```python
from build123d import *

# Parameters (mm, degrees)
SKETCH2_R           = 1.5
BOSS_EXTRUDE1_DEPTH = 45
CHAMFER1_SIZE       = 0.3
SKETCH6_W           = 3
SKETCH6_H           = 2.75
CUT_EXTRUDE1_DEPTH  = 1.6
SKETCH8_R           = 1.493375673
CUT_EXTRUDE2_DEPTH  = 1
CUT_EXTRUDE2_TAPER  = 45


with BuildPart() as part:
    # Sketch2 → Boss-Extrude1 (new body)
    with BuildSketch(Plane(origin=(0, 0, 0), x_dir=(0, 0, -1), z_dir=(1, 0, 0))):
        Circle(SKETCH2_R)
    extrude(amount=-BOSS_EXTRUDE1_DEPTH)

    # Chamfer1
    chamfer1_edges = [part.edges().sort_by_distance(p)[0] for p in [
        (0, 0, 1.5),
    ]]
    chamfer(chamfer1_edges, length=CHAMFER1_SIZE)

    # Sketch6 → Revolve1 (revolve)
    with BuildSketch(Plane.XY):
        with Locations((-46.5, 1.375)):
            Rectangle(SKETCH6_W, SKETCH6_H)
    revolve(axis=Axis((-45, 0, 0), (1, 0, 0)))

    # Sketch7 → Cut-Extrude1 (cut)
    with BuildSketch(Plane.ZY.offset(48)):
        Polygon((0, 1.443375673), (-1.25, 0.721687836), (-1.25, -0.721687836), (0, -1.443375673), (1.25, -0.721687836), (1.25, 0.721687836), align=None)
    extrude(amount=-CUT_EXTRUDE1_DEPTH, mode=Mode.SUBTRACT)

    # Sketch8 → Cut-Extrude2 (cut)
    with BuildSketch(Plane.ZY.offset(48)):
        Circle(SKETCH8_R)
    extrude(amount=-CUT_EXTRUDE2_DEPTH, taper=CUT_EXTRUDE2_TAPER, mode=Mode.SUBTRACT)


solid = part.part
```
The listing builds one solid part. Answer for the finished solid, in the listing's coordinates (mm). A direction names the side the tool comes from. Coordinates: 2 decimals unless noted, no trailing zeros. Loops run counter-clockwise (first coordinate to the right, second up) from the corner with the lowest first, then second, coordinate; pieces in that order, holes last. Notation, with made-up numbers: (8.25, -39.5) -> (28.25, -39.5) arc R22 cw to (28.25, -31.5) -> close; hole circle Ø6 at (45, -13.75). An arc over 180 degrees is marked (long way). Return JSON: item names as keys, results as strings. Group by question number.
(1) Determine the mould class of faces 1 (the cylindrical face through (-46.479, -0.596, -2.685)), 2 (the flat face through (-46.4, 0, 0)), 3 (the flat face through (-48, -1.2, -1.2)) for opening direction Y: released by +Y, released by -Y, zero draft, split by the parting line, or undercut.
(2) Which of the six approach directions +Z, -Z, +X, -X, +Y, -Y give full straight-line access (tool end or side, diameter ignored) to faces 4 (the flat face through (-45, -1.2, -1.2)), 5 (the flat face through (0, 0, 0)), 6 (the flat face through (-47, 0, 1.25))?
(3) A cutting plane is placed at A-A on z = 2.05. Write down the section's boundary in (x, y), and give its area (3 significant figures).
(4) A cutting plane is placed at B-B on x = -16. Write down the section's boundary in (y, z), and give its area (3 significant figures).
(5) Find the intervals of material crossed by probe 1 along X at (y, z) = (0.25, -2.2); probe 2 along Y at (x, z) = (-11, 0.15); probe 3 along Y at (x, z) = (-25, -0.4), in increasing order. Write a range as from..to.
(6) A cutting plane is placed at C-C on z = -2.1. Write down the section's boundary in (x, y), and give its area (3 significant figures).
(7) Given pin 1 Ø3 at (x, z) = (-22, -1) entering from +Y; pin 2 Ø1.5 at (x, z) = (-27.5, 2) entering from +Y; pin 3 Ø1.5 at (x, z) = (-29, 0) entering from -Y, each flat-ended and moving along its own axis, determine where each tip first touches the part or whether it passes through.
The answers:
{
 "1": {"face 1": "split by the parting line", "face 2": "undercut", "face 3": "zero draft"},
 "2": {"face 4": "+X", "face 5": "+Z, -Z, +X, +Y, -Y", "face 6": "-X"},
 "3": {"outline": "(-48, -1.83) -> (-45, -1.83) -> (-45, 1.83) -> (-48, 1.83) -> close", "area": "11.0 mm^2"},
 "4": {"outline": "circle Ø3 at (0, 0)", "area": "7.07 mm^2"},
 "5": {"probe 1": "x = -48..-45", "probe 2": "y = -1.49..1.49", "probe 3": "y = -1.45..1.45"},
 "6": {"outline": "(-48, -1.78) -> (-45, -1.78) -> (-45, 1.78) -> (-48, 1.78) -> close", "area": "10.7 mm^2"},
 "7": {"pin 1": "stops at y = 1.5", "pin 2": "stops at y = 0.83", "pin 3": "stops at y = -1.5"}
}
